from build123d import *

# Parameters (mm, degrees)
SKETCH2_W               = 200
SKETCH2_H               = 225
BOSS_EXTRUDE1_DEPTH     = 4.7625
M5_CLEARANCE_HOLE1_D    = 5.3
F_1_4_CLEARANCE_HOLE1_D = 6.5278
CUT_EXTRUDE1_DEPTH      = 151.595256918
F_1_4_CLEARANCE_HOLE2_D = 6.5278
FILLET1_R               = 2
FILLET2_R               = 3


with BuildPart() as part:
    # Sketch2 → Boss-Extrude1 (new body)
    with BuildSketch(Plane(origin=(0, 0, 0), x_dir=(1, 0, 0), z_dir=(0, 1, 0))):
        Rectangle(SKETCH2_W, SKETCH2_H)
    extrude(amount=BOSS_EXTRUDE1_DEPTH)

    # M5 Clearance Hole1 (through all)
    with Locations(Plane(origin=(0, 4.7625, 0), x_dir=(1, 0, 0), z_dir=(0, 1, 0))):
        with Locations((-95, 62.5), (-95, -62.5), (95, -62.5), (95, 62.5)):
            Hole(M5_CLEARANCE_HOLE1_D / 2)

    # 1/4 Clearance Hole1 (through all)
    with Locations(Plane(origin=(0, 4.7625, 0), x_dir=(1, 0, 0), z_dir=(0, 1, 0))):
        with Locations((0, 100), (-90, -100), (90, -100)):
            Hole(F_1_4_CLEARANCE_HOLE1_D / 2)

    # Sketch7 → Cut-Extrude1 (cut, through all)
    with BuildSketch(Plane(origin=(0, 4.7625, 0), x_dir=(1, 0, 0), z_dir=(0, 1, 0))):
        Polygon((-82.788897449, 60), (82.788897449, 60), (0, 4.807401701), align=None)
        Polygon((-90, 55.192598299), (-7.211102551, 0), (-90, -55.192598299), align=None)
        Polygon((90, 55.192598299), (7.211102551, 0), (90, -55.192598299), align=None)
        Polygon((-82.788897449, -60), (0, -4.807401701), (82.788897449, -60), align=None)
        Polygon((-80, -74.081685467), (-20.094451529, -86.25), (-80, -98.418314533), align=None)
        Polygon((-59.905548471, -70), (59.905548471, -70), (0, -82.168314533), align=None)
        Polygon((80, -74.081685467), (20.094451529, -86.25), (80, -98.418314533), align=None)
        Polygon((-59.905548471, -102.5), (0, -90.331685467), (59.905548471, -102.5), align=None)
        Polygon((90, 98.18252099), (60.627640639, 86.25), (90, 74.31747901), align=None)
        Polygon((79.372359361, 102.5), (50, 90.56747901), (20.627640639, 102.5), align=None)
        Polygon((10, 98.18252099), (39.372359361, 86.25), (10, 74.31747901), align=None)
        Polygon((20.627640639, 70), (50, 81.93252099), (79.372359361, 70), align=None)
        Polygon((-79.372359361, 102.5), (-20.627640639, 102.5), (-50, 90.56747901), align=None)
        Polygon((-10, 98.18252099), (-39.372359361, 86.25), (-10, 74.31747901), align=None)
        Polygon((-50, 81.93252099), (-79.372359361, 70), (-20.627640639, 70), align=None)
        Polygon((-90, 74.31747901), (-60.627640639, 86.25), (-90, 98.18252099), align=None)
    extrude(amount=-CUT_EXTRUDE1_DEPTH, mode=Mode.SUBTRACT)

    # 1/4 Clearance Hole2 (through all)
    with Locations(Plane(origin=(0, 4.7625, 0), x_dir=(1, 0, 0), z_dir=(0, 1, 0))):
        with Locations((0, -86.25), (-90, 104.5), (90, 104.5)):
            Hole(F_1_4_CLEARANCE_HOLE2_D / 2)

    # Fillet1
    fillet1_edges = [part.edges().sort_by_distance(p)[0] for p in [
        (-80, 2.38125, 98.418314533),
        (-80, 2.38125, 74.081685467),
        (-20.094451529, 2.38125, 86.25),
        (80, 2.38125, 74.081685467),
        (80, 2.38125, 98.418314533),
        (20.094451529, 2.38125, 86.25),
        (59.905548471, 2.38125, 102.5),
        (-59.905548471, 2.38125, 102.5),
        (0, 2.38125, 90.331685467),
        (90, 2.38125, -98.18252099),
        (90, 2.38125, -74.31747901),
        (60.627640639, 2.38125, -86.25),
        (-90, 2.38125, 55.192598299),
        (-90, 2.38125, -55.192598299),
        (-7.211102551, 2.38125, 0),
        (90, 2.38125, -55.192598299),
        (90, 2.38125, 55.192598299),
        (7.211102551, 2.38125, 0),
        (82.788897449, 2.38125, 60),
        (-82.788897449, 2.38125, 60),
        (0, 2.38125, 4.807401701),
        (0, 2.38125, 82.168314533),
        (-59.905548471, 2.38125, 70),
        (59.905548471, 2.38125, 70),
        (-50, 2.38125, -81.93252099),
        (-20.627640639, 2.38125, -70),
        (-79.372359361, 2.38125, -70),
        (-10, 2.38125, -98.18252099),
        (-10, 2.38125, -74.31747901),
        (-39.372359361, 2.38125, -86.25),
        (-90, 2.38125, -74.31747901),
        (-90, 2.38125, -98.18252099),
        (-60.627640639, 2.38125, -86.25),
        (20.627640639, 2.38125, -102.5),
        (79.372359361, 2.38125, -102.5),
        (50, 2.38125, -90.56747901),
        (10, 2.38125, -74.31747901),
        (10, 2.38125, -98.18252099),
        (39.372359361, 2.38125, -86.25),
        (79.372359361, 2.38125, -70),
        (20.627640639, 2.38125, -70),
        (50, 2.38125, -81.93252099),
        (-50, 2.38125, -90.56747901),
        (-79.372359361, 2.38125, -102.5),
        (-20.627640639, 2.38125, -102.5),
        (0, 2.38125, -4.807401701),
        (-82.788897449, 2.38125, -60),
        (82.788897449, 2.38125, -60),
    ]]
    fillet(fillet1_edges, radius=FILLET1_R)

    # Fillet2
    fillet2_edges = [part.edges().sort_by_distance(p)[0] for p in [
        (100, 2.38125, 112.5),
        (-100, 2.38125, 112.5),
        (-100, 2.38125, -112.5),
        (100, 2.38125, -112.5),
    ]]
    fillet(fillet2_edges, radius=FILLET2_R)


solid = part.part
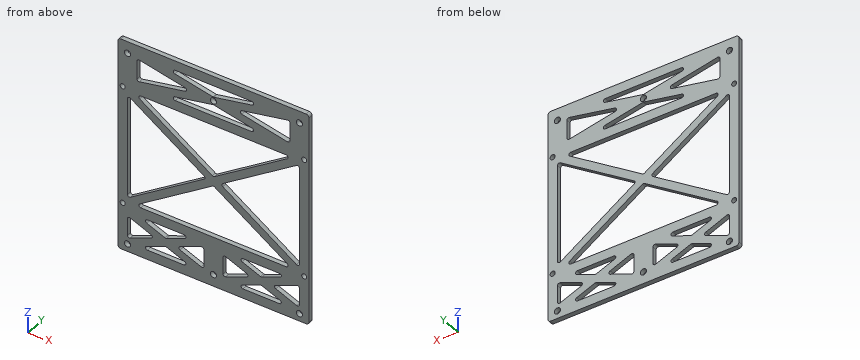
Geometry: final body of the model. Coordinates: model frame, mm. Give positions to 0.01 mm unless a question says otherwise; leave off trailing zeros. Order: outer loops, then holes, each group sorted by start corner. A loop starts at its lowest first (then second) coordinate and runs counter-clockwise, first axis right, second up. Notation, with made-up numbers: (41.25, 42.25) - (76.25, 42.25) arc R23 cw to (76.25, 57.25) - close; hole circle Ø11 at (42.25, -35). An arc over 180 degrees is marked (long way). Use CSV: the item, a comma, the result in double quotes.
1. Section query B-B (y = 3.7). Give the number of separate pieces and of enclosed holes in the cut face, plus the area to 3 significant figures.
Answers below:
separate pieces,"1"
enclosed holes,"26"
area,"21,100 mm2"
2. Section query A-A (z = 62.5). Output: boundary loops of the cut face in (x, y).
Answers below:
outline,"(-100, 0) - (-97.65, 0) - (-97.65, 4.76) - (-100, 4.76) - close; (-92.35, 0) - (92.35, 0) - (92.35, 4.76) - (-92.35, 4.76) - close; (97.65, 0) - (100, 0) - (100, 4.76) - (97.65, 4.76) - close"
3. Material intervals for line 1 along Z through (x, y) = (95, 3.15); line 2 along X through (y, z) = (1.3, -62.5); line 3 along X through (y, z) = (3.5, -104.5), sorted ascending. Write a range as from..to.
Answers below:
line 1,"-112.5..-65.15, -59.85..59.85, 65.15..112.5"
line 2,"-100..-97.65, -92.35..92.35, 97.65..100"
line 3,"-100..-93.26, -86.74..86.74, 93.26..100"
